Autodesk Fusion 360 part; units mm, degrees
sketch "Sketch1" plane through (0, 0, 0) normal (0, 0, 1) x (1, 0, 0)
  line L0 (25.455, -18.47) -> (-25.455, -18.47)
  line L1 (-25.455, -18.47) -> (-25.455, 18.47)
  line L2 (-25.455, 18.47) -> (25.455, 18.47)
  line L3 (25.455, 18.47) -> (25.455, -18.47)
  line L4 (25.455, -18.47) -> (-25.455, 18.47) construction
  line L5 (-25.455, -18.47) -> (25.455, 18.47) construction
  circle A0 centre (20.955, 13.97) radius 4.5
  circle A1 centre (20.955, 13.97) radius 2.55
  line L6 (0, 1.75) -> (0, 22.5)
  circle A2 centre (-20.955, 13.97) radius 2.55
  circle A3 centre (-20.955, 13.97) radius 4.5
  line L7 (1.75, 0) -> (22.5, 0)
  circle A4 centre (20.955, -13.97) radius 4.5
  circle A5 centre (20.955, -13.97) radius 2.55
  circle A6 centre (-20.955, -13.97) radius 4.5
  circle A7 centre (-20.955, -13.97) radius 2.55
  dimension "d8" = 5.1
  dimension "d9" = 9
  dimension "d10" = 41.91
  dimension "d11" = 27.94
extrude "Extrude1" add sketch "Sketch1" against normal blind 5 contours L0 L1 L2 L3 A0 A3 A4 A6 | A4 | A6 | A0 | A3 | A1 | A2 | A5 | A7
extrude "Extrude2" add sketch "Sketch1" along normal blind 6 contours A4 | A6 | A0 | A3 | A1 | A2 | A5 | A7
extrude "Extrude3" cut sketch "Sketch1" against normal blind 7 from surface at 6 contours A1 | A2 | A5 | A7
Verification items for the finished model (mm, model axes). A direction names the side the tool comes from. Coordinates: 2 decimals unless noted, no trailing zeros. Loops run counter-clockwise (first coordinate to the right, second up) from the corner with the lowest first, then second, coordinate; pieces in that order, holes last. Notation, with made-up numbers: (5, 48) - (41, 48) arc R29 ccw to (41, 68) - close; hole circle Ø8 at (80, 38.5). An arc over 180 degrees is marked (long way). Return JSON: item names as keys, results as strings.
1. Go/stop test with flat-tipped pins: pin 1 (5.5 mm diameter, centred on x = 20.5, y = 14, fed in from +Z); pin 2 (6 mm diameter, centred on x = -5, z = 4.5, fed in from -Y); pin 3 (2.5 mm diameter, centred on x = -22, y = -14.5, fed in from +Z). Record where each tip stops, or that it passes through.
Established:
{"pin 1": "stops at z = 6", "pin 2": "passes through", "pin 3": "stops at z = -1"}
2. Thickness scan on L1, parallel to Y at x = -22, z = 2.5; L2, parallel to Z at x = 18, y = 10.5; L3, parallel to Y at x = -18, z = 5.5. Record the ranges inside material, lowest first.
Established:
{"L1": "y = -18.35 to -16.3, -11.64 to -9.59, 9.59 to 11.64, 16.3 to 18.35", "L2": "z = -5 to 0", "L3": "y = -17.36 to -10.58, 10.58 to 17.36"}
3. Section check D-D, the plane y = 4.5. Record the boundary of the cut face in (x, z) (3 decimals), then the cut area to 3 significant figures.
Established:
{"outline": "(-25.455, -5) - (25.455, -5) - (25.455, 0) - (-25.455, 0) - close", "area": "255 mm2"}
4. Section check C-C, the plane x = -19.5. Record the boundary of the cut face in (y, z), then the cut area to 3 significant figures.
Established:
{"outline": "(-18.47, -5) - (18.47, -5) - (18.47, 0) - (18.23, 0) - (18.23, 6) - (16.06, 6) - (16.06, -1) - (11.88, -1) - (11.88, 6) - (9.71, 6) - (9.71, 0) - (-9.71, 0) - (-9.71, 6) - (-11.88, 6) - (-11.88, -1) - (-16.06, -1) - (-16.06, 6) - (-18.23, 6) - (-18.23, 0) - (-18.47, 0) - close", "area": "228 mm2"}
5. Tool access check on faces 1 (the cylindrical face through (18.93, -15.52, 2.55)), 2 (the flat face through (-25.455, 0, -2)). Record the directions out of +Z, -Z, +X, -X, +Y, -Y that give a thin tool (end or side, any length) a straight path to the whole face; none if there is none.
Established:
{"face 1": "+Z", "face 2": "+Z, -Z, -X, +Y, -Y"}
6. Mould release check, pull along X, two halves, no side actions. Record for faces 3 (the cylindrical face through (-24.272, 17.011, 1.799)), 4 (the flat face through (25.455, 0, -2)), 5 (the flat face through (23, -16, 6)): +X half, -X half, draft (parallel to the pull), parting line (faces both ways), or undercut.
Established:
{"face 3": "undercut", "face 4": "+X half", "face 5": "draft"}
7. Section check B-B, the plane y = -15. Record the boundary of the cut face in (x, z).
Established:
{"outline": "(-25.34, -5) - (25.34, -5) - (25.34, 6) - (23.29, 6) - (23.29, -1) - (18.62, -1) - (18.62, 6) - (16.57, 6) - (16.57, 0) - (-16.57, 0) - (-16.57, 6) - (-18.62, 6) - (-18.62, -1) - (-23.29, -1) - (-23.29, 6) - (-25.34, 6) - close"}
8. Section check A-A, the plane z = 2.5. Record the boundary of the cut face in (x, y) (3 decimals).
Established:
{"outline": "circle Ø9 at (-20.955, -13.97); circle Ø9 at (-20.955, 13.97); circle Ø9 at (20.955, -13.97); circle Ø9 at (20.955, 13.97); hole circle Ø5.1 at (-20.955, -13.97); hole circle Ø5.1 at (-20.955, 13.97); hole circle Ø5.1 at (20.955, -13.97); hole circle Ø5.1 at (20.955, 13.97)"}
